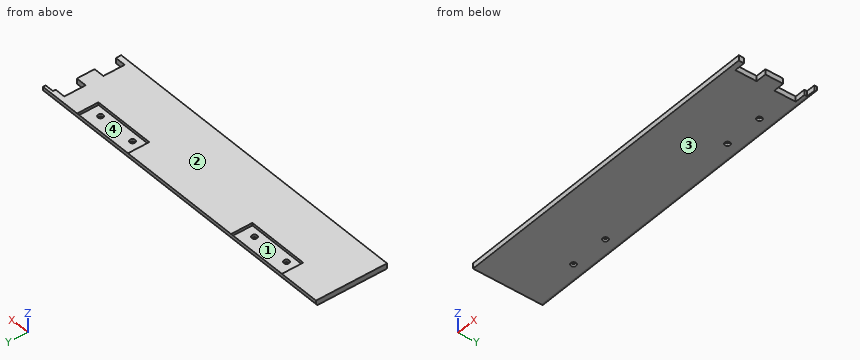
from build123d import *

# Parameters (mm, degrees)
ESQUISSE1_W             = 188
ESQUISSE1_H             = 40
BOSS_EXTRU_1_DEPTH      = 3
CONG_3_R                = 1.5
ENL_V_MAT_EXTRU_1_DEPTH = 193.231631112
ESQUISSE5_W             = 35
ESQUISSE5_H             = 12
ENL_V_MAT_EXTRU_2_DEPTH = 1.5
ESQUISSE7_R             = 1.5
ENL_V_MAT_EXTRU_3_DEPTH = 1.5
ESQUISSE8_R             = 1.5
ENL_V_MAT_EXTRU_4_DEPTH = 1.5


with BuildPart() as part:
    # Esquisse1 → Boss.-Extru.1 (new body)
    with BuildSketch(Plane.XY):
        with Locations((94, 20)):
            Rectangle(ESQUISSE1_W, ESQUISSE1_H)
    extrude(amount=BOSS_EXTRU_1_DEPTH)

    # Congé3
    cong_3_edges = [part.edges().sort_by_distance(p)[0] for p in [
        (94, 40, 0),
    ]]
    fillet(cong_3_edges, radius=CONG_3_R)

    # Esquisse3 → Enlèv. mat.-Extru.1 (cut, through all)
    with BuildSketch(Plane(origin=(0, 0, 0), x_dir=(-1, 0, 0), z_dir=(0, 0, -1))):
        Polygon((-177, 37), (-183, 37), (-183, 38.5), (-188, 38.5), (-188, 0), (-183, 0), (-183, 3), (-177, 3), (-177, 15), (-183, 15), (-183, 25), (-177, 25), align=None)
    extrude(amount=-ENL_V_MAT_EXTRU_1_DEPTH, mode=Mode.SUBTRACT)

    # Esquisse5 → Enlèv. mat.-Extru.2 (cut)
    with BuildSketch(Plane.XY.offset(3)):
        with Locations((147, 33.99)):
            Rectangle(ESQUISSE5_W, ESQUISSE5_H)
        with Locations((41, 33.99)):
            Rectangle(ESQUISSE5_W, ESQUISSE5_H)
    extrude(amount=-ENL_V_MAT_EXTRU_2_DEPTH, mode=Mode.SUBTRACT)

    # Esquisse7 → Enlèv. mat.-Extru.3 (cut)
    with BuildSketch(Plane.XY.offset(1.5)):
        with Locations((30, 32.1)):
            Circle(ESQUISSE7_R)
        with Locations((52, 32.1)):
            Circle(ESQUISSE7_R)
    extrude(amount=-ENL_V_MAT_EXTRU_3_DEPTH, mode=Mode.SUBTRACT)

    # Esquisse8 → Enlèv. mat.-Extru.4 (cut)
    with BuildSketch(Plane.XY.offset(1.5)):
        with Locations((136, 32.1)):
            Circle(ESQUISSE8_R)
        with Locations((158, 32.1)):
            Circle(ESQUISSE8_R)
    extrude(amount=-ENL_V_MAT_EXTRU_4_DEPTH, mode=Mode.SUBTRACT)


solid = part.part
Verification items for the finished model (mm, model axes). Face numbers are marked on the shaded views. A direction names the side the tool comes from. Coordinates: 2 decimals unless noted, no trailing zeros. Order: outer loops, then holes, each group sorted by start corner. A loop starts at its lowest first (then second) coordinate and runs counter-clockwise, first axis right, second up. Notation, with made-up numbers: M 15,49.5 L 32,49.5 A5 cw 32,56.5 Z; hole C -17.5,30.25 d11. An arc over 180 degrees is marked long. One line per item, written item: value. Start each with the question number.
Item 1: Sectioned sample at C-C on y = 7.5. Record the cut outline in (x, z).
Item 2: Thickness scan on probe 1 along X at (y, z) = (30.5, 2.8); probe 2 along Y at (x, z) = (158, 1.15); probe 3 along X at (y, z) = (34.5, 1.4). Record the ranges inside material, lowest first.
Item 3: Mould release check, pull along Y, two halves, no side actions. Record for the marked faces 3 and 4: pulls with the +Y half, pulls with the -Y half, needs draft (parallel to the pull), parting line crosses it, or undercut.
Item 4: Access from +Z, -Z, +X, -X, +Y, -Y to the whole of each face (thin tool, end or side, straight path). Record for the marked faces 1 and 2.
Item 5: Sectioned sample at A-A on z = 2.4. Record the cut outline in (x, y).
Item 6: Depth check by flat-ended pin: P1, Ø9.5, axis at x = 146, y = 33, coming from the +Z side; P2, Ø1.2, axis at y = 35.5, z = 2, coming from the +X side; P3, Ø2.5, axis at x = 136, y = 32.1, coming from the -Z side. Enter the tip coordinate at first touch or a pass-through.
Calculated:
1. outline: M 0,0 L 177,0 L 177,3 L 0,3 Z
2. probe 1: 0 to 23.5, 58.5 to 129.5, 164.5 to 177
2. probe 2: 0 to 30.6, 33.6 to 39.96
2. probe 3: 0 to 177
3. face 3: needs draft
3. face 4: undercut
4. face 1: +Z
4. face 2: +Z, +X, -X, +Y, -Y
5. outline: M 0,0 L 183,0 L 183,3 L 177,3 L 177,15 L 183,15 L 183,25 L 177,25 L 177,37 L 183,37 L 183,38.5 L 188,38.5 L 188,40 L 0,40 Z; hole M 23.5,27.99 L 58.5,27.99 L 58.5,39.99 L 23.5,39.99 Z; hole M 129.5,27.99 L 164.5,27.99 L 164.5,39.99 L 129.5,39.99 Z
6. P1: z = 1.5
6. P2: x = 177
6. P3: through
